Could you check a few things on this model? Use its own coordinates, in mm. A direction names the side the tool comes from. Round coordinates to 2 decimals unless told otherwise and drop trailing zeros. Loops run counter-clockwise (first coordinate to the right, second up) from the corner with the lowest first, then second, coordinate; pieces in that order, holes last. Notation, with made-up numbers: (19.5, -32) -> (69.5, -32) arc R15 cw to (69.5, -18) -> close; hole circle Ø5 at (9, -30.75). An arc over 180 degrees is marked (long way). Put each result on its own line as item: value. Start each with the question number.
1. Which directions (+Z, -Z, +X, -X, +Y, -Y) give clear straight access to the entire face, cutting with the end or side of a thin tool? Please do faces 4 (the flat face through (-5.3, 2, -4)), 5 (the cylindrical face through (4.07, 1.28, 2.83)), 6 (the flat face through (-0.1, -6.3, -0.8)).
2. Imagine slicing it at A-A, the plane z = -3.5. Please give me the cut outline in (x, y).
3. I'm going to push flat-ended pins straight in: P1, Ø5, axis at x = -3, z = -2.5, coming from the +Y side; P2, Ø3, axis at x = -2.5, z = 3.5, coming from the -Y side; P3, Ø8, axis at y = -0.5, z = -1.5, coming from the +X side; P4, Ø3, axis at y = 5.5, z = -4.5, coming from the -X side. Where does each tip first touch, or does it pass through?
4. I need wall thicknesses on line 1 (X direction, y = 1.75, z = -5.5); line 2 (Z direction, x = -3, y = 0); line 3 (Z direction, x = -0.25, y = 0). Which ranges of each line are inside material? Lowest first, please. Write a range as [from, to].
5. Imagine slicing it at B-B, the plane z = 2.5. Please give me the cut outline in (x, y), and give its area (3 significant figures).
6. If we mould it in two halves opening along Z, with no side actions, what happens to faces 1 (the flat face through (0, -8.1, -6)), 2 (the flat face through (0, 0, -9)), 3 (the cylindrical face through (0, 0, -2))? For each: pulls with the +Z half, pulls with the -Z half, needs draft (parallel to the pull), parting line crosses it, or undercut.
```python
from build123d import *

# Parameters (mm, degrees)
F2_W          = 10.6
F2_H          = 16.2
F3_DEPTH      = 1
F3_DEPTH_BACK = 9
F4_R          = 1.5
F5_DEPTH      = 10.6
F6_SIZE       = 3.6
F7_R          = 2.5


with BuildPart() as f1:
    # F0 (on Front) → F1 (revolve)
    with BuildSketch(Plane.XZ):
        with BuildLine():
            Line((4.264979, 0), (4.264979, 5.628212))
            ThreePointArc((4.264979, 5.628212), (5.979107, 12.682604), (0, 16.8))
            Line((0, 16.8), (0, 0))
            Line((0, 0), (4.264979, 0))
        make_face()
    revolve(axis=Axis((0, 0, 30.748535), (0, 0, 1)))

    # F2 (on Top) → F3 (join, two sides)
    with BuildSketch(Plane.XY) as f3_sk:
        Rectangle(F2_W, F2_H)
    extrude(amount=F3_DEPTH)
    extrude(f3_sk.sketch, amount=-F3_DEPTH_BACK)

    # F4 (on face) → F5 (cut, through all)
    with BuildSketch(Plane.YZ.offset(5.3)):
        with Locations((0, -3.5)):
            Circle(F4_R)
    extrude(amount=-F5_DEPTH, mode=Mode.SUBTRACT)

    # F6
    f6_edges = [f1.edges().sort_by_distance(p)[0] for p in [
        (0, 8.1, 1),
        (0, -8.1, 1),
    ]]
    chamfer(f6_edges, length=F6_SIZE)

    # F7
    f7_edges = [f1.edges().sort_by_distance(p)[0] for p in [
        (-4.264979, 0, 5.628212),
    ]]
    fillet(f7_edges, radius=F7_R)


solid = f1.part
```
Entries:
1. face 4: -Z, -X, +Y, -Y
1. face 5: none
1. face 6: +X, -X, -Y
2. outline: (-5.3, -8.1) -> (5.3, -8.1) -> (5.3, -1.5) -> (-5.3, -1.5) -> close; (-5.3, 1.5) -> (5.3, 1.5) -> (5.3, 8.1) -> (-5.3, 8.1) -> close
3. P1: y = 8.1
3. P2: y = -4.15
3. P3: x = 5.3
3. P4: x = -5.3
4. line 1: [-5.3, 5.3]
4. line 2: [-9, -5], [-2, 16.05]
4. line 3: [-9, -5], [-2, 16.8]
5. outline: circle Ø8.53 at (0, 0)
5. area: 57.1 mm^2
6. face 1: needs draft
6. face 2: pulls with the -Z half
6. face 3: undercut
